```python
from build123d import *

# Parameters (mm, degrees)
F0_R      = 20
F1_DEPTH  = 16
F2_W      = 10
F2_H      = 20
F3_DEPTH  = 9
F4_W      = 4.5
F4_H      = 2
F5_DEPTH  = 7.001
F7_R      = 4
F7_R_2    = 3.8
F8_DEPTH  = 12.8
F10_DEPTH = 11.7


with BuildPart() as f1:
    # F0 (on Top) → F1 (new body)
    with BuildSketch(Plane.XY):
        Circle(F0_R)
    extrude(amount=F1_DEPTH)

    # F2 (on face) → F3 (cut)
    with BuildSketch(Plane(origin=(0, 0, 0), x_dir=(1, 0, 0), z_dir=(0, 0, -1))):
        Rectangle(F2_W, F2_H)
    extrude(amount=-F3_DEPTH, mode=Mode.SUBTRACT)

    # F4 (on face) → F5 (cut, through all)
    with BuildSketch(Plane(origin=(0, 0, 9), x_dir=(1, 0, 0), z_dir=(0, 0, -1))):
        with Locations((0, 9)):
            Rectangle(F4_W, F4_H)
        with Locations((0, -9)):
            Rectangle(F4_W, F4_H)
    extrude(amount=-F5_DEPTH, mode=Mode.SUBTRACT)

    # F7 (on offset) → F8 (cut)
    with BuildSketch(Plane.XY.offset(14)):
        with Locations((-13.818456, 0)):
            Circle(F7_R)
        with Locations((-13.818456, 0)):
            Circle(F7_R_2, mode=Mode.SUBTRACT)
    extrude(amount=-F8_DEPTH, mode=Mode.SUBTRACT)

    # F9 (on offset) → F10 (cut)
    with BuildSketch(Plane.XY.offset(14)):
        with BuildLine():
            Line((-26.818456, -6.657433), (-16.5516, -2.920603))
            ThreePointArc((-16.5516, -2.920603), (-9.818456, 0), (-16.5516, 2.920603))
            Line((-16.5516, 2.920603), (-26.818456, 6.657433))
            Line((-26.818456, 6.657433), (-26.818456, 0))
            Line((-26.818456, 0), (-26.818456, -6.657433))
        make_face()
    extrude(amount=-F10_DEPTH, mode=Mode.SUBTRACT)


solid = f1.part
```
Can you work these out from the model? Positions are in its coordinate system, mm. A direction names the side the tool comes from. Give positions to 0.01 mm unless a question says otherwise; leave off trailing zeros. Write each loop counter-clockwise with the first axis right and the second up, starting at its lowest first coordinate (ties: lowest second). Pieces come first, ordered by that corner, then holes. Notation, with made-up numbers: (-3.5, 31) - (15.5, 31) arc R26 ccw to (15.5, 51) - close; hole circle Ø1 at (17, 54). An arc over 180 degrees is marked (long way). Write item = value, one per line. Start each with the question number.
1. Imagine slicing it at C-C (z = 7.75). Please give me the cut outline in (x, y).
2. Imagine slicing it at A-A (z = 12.5). Please give me the cut outline in (x, y).
3. Thinking about a two-plate mould opening in Z: for faces 5 (the face through (-5, 0, 4)), 6 (the face through (-18.09, -3.48, 8.23)), 7 (the face through (9, 0, 0)), which applies, released by +Z, released by -Z, zero draft, split by the parting line, or undercut?
4. For pin 1 (9 mm diameter, centred on x = -13.5, y = -0.5, fed in from -Z); pin 2 (4 mm diameter, centred on y = 2.5, z = 11, fed in from -X); pin 3 (0.6 mm diameter, centred on y = 9, z = 11.5, fed in from +X); pin 4 (8 mm diameter, centred on x = 12.5, z = 9.5, fed in from +Y), each with a flat end and sliding along its axis, tell me the tip position at first contact or that it passes through.
5. Please list where these lines run through material, in increasing order: line 1 (X direction, y = 0, z = 6.5); line 2 (Y direction, x = 1.5, z = 10.5); line 3 (X direction, y = -6.5, z = 8).
6. Imagine slicing it at D-D (y = 0). Please give me the cut outline in (x, z), and give its area (3 significant figures).
7. On a 3-axis mill with a long thin cutter (end or side, diameter ignored), from which of +Z, -Z, +X, -X, +Y, -Y can I reach the whole of each face in a straight line? I mean faces 1 (the face through (0, -10, 6)), 2 (the face through (2.25, -9, 12)), 3 (the face through (-10.123, -1.532, 7.69)), 4 (the face through (-18.05, 3.466, 8.232)). Say none if no direction works.
8. Imagine slicing it at B-B (x = 0). Please give me the cut outline in (y, z).
Worked answers:
q1.outline = (-19.59, -4.03) arc R20 ccw (long way) to (-19.59, 4.03) - (-16.55, 2.92) arc R4 cw (long way) to (-16.55, -2.92) - close; hole (-5, -10) - (5, -10) - (5, 10) - (-5, 10) - close
q2.outline = (-19.59, -4.03) arc R20 ccw (long way) to (-19.59, 4.03) - (-16.55, 2.92) arc R4 cw (long way) to (-16.55, -2.92) - close; hole (-2.25, -10) - (2.25, -10) - (2.25, -8) - (-2.25, -8) - close; hole (-2.25, 8) - (2.25, 8) - (2.25, 10) - (-2.25, 10) - close
q3.face_5 = zero draft
q3.face_6 = undercut
q3.face_7 = released by -Z
q4.pin_1 = 0
q4.pin_2 = -19.59
q4.pin_3 = 18.01
q4.pin_4 = 18.1
q5.line_1 = -9.82 to -5, 5 to 20
q5.line_2 = -19.94 to -10, -8 to 8, 10 to 19.94
q5.line_3 = -18.91 to -5, 5 to 18.91
q6.outline = (-20, 0) - (-5, 0) - (-5, 9) - (5, 9) - (5, 0) - (20, 0) - (20, 16) - (-20, 16) - (-20, 14) - (-9.82, 14) - (-9.82, 1.2) - (-10.02, 1.2) - (-10.02, 2.3) - (-17.62, 2.3) - (-17.62, 1.2) - (-17.82, 1.2) - (-17.82, 2.3) - (-20, 2.3) - close
q6.area = 430 mm2
q7.face_1 = -Z
q7.face_2 = +Z, -Z
q7.face_3 = none
q7.face_4 = -X
q8.outline = (-20, 0) - (-10, 0) - (-10, 16) - (-20, 16) - close; (-8, 9) - (8, 9) - (8, 16) - (-8, 16) - close; (10, 0) - (20, 0) - (20, 16) - (10, 16) - close
